Geometry: final body of the model. Coordinates: model frame, mm. Face numbers are marked on the shaded views. A direction names the side the tool comes from. Coordinates: 2 decimals unless noted, no trailing zeros. Write each loop counter-clockwise with the first axis right and the second up, starting at its lowest first coordinate (ties: lowest second). Pieces come first, ordered by that corner, then holes. Notation, with made-up numbers: (77, 56) - (87, 56) arc R9 cw to (87, 62) - close; hole circle Ø9 at (-27, 14.25). An arc over 180 degrees is marked (long way). Answer as a JSON object with one key per item and string values. Group by question number.
Item 1: Section D-D on y = -7.5. Return loops of the section in (x, z).
Item 2: Set-up query: the marked faces 1, 2 and 3. Return all of +Z, -Z, +X, -X, +Y, -Y with unobstructed straight access to the full face (end or side cutting, diameter ignored); none if empty.
Item 3: First-contact query: pin 1 Ø1 at (x, y) = (23.5, -0.5) entering from +Z; pin 2 Ø1 at (x, z) = (0, 5.5) entering from +Y; pin 3 Ø3.5 at (y, z) = (8.5, 3) entering from +X. Flat tips, straight axial feed; report the tip coordinate or a pass-through.
Item 4: Section A-A on y = 25.5. Return loops of the section in (x, z), and give its area (3 significant figures).
Item 5: Line query: line 1 along Z through (x, y) = (-2, -27); line 2 along Z through (x, y) = (6.5, 10.5); line 3 along X through (y, z) = (2.5, 8.5). Output: solid intervals per line, ascending. Write a range as from..to.
Item 6: Section B-B on z = 3.5. Return loops of the section in (x, y), and give its area (3 significant figures).
Item 7: Section C-C on x = -2.5. Return loops of the section in (y, z).
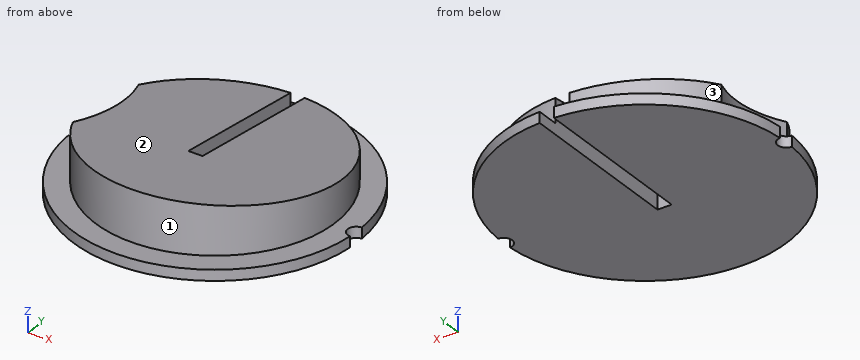
```python
from build123d import *

# Parameters (mm, degrees)
F1_DEPTH = 2.413
F3_DEPTH = 25.4
F5_DEPTH = 31.75
F7_DEPTH = 25.4


with BuildPart() as f1:
    # F0 (on Top) → F1 (new body)
    with BuildSketch(Plane.XY):
        with BuildLine():
            ThreePointArc((31.629235, -1.904139), (29.7815, 0), (31.629235, 1.904139))
            ThreePointArc((31.629235, 1.904139), (0, 31.6865), (-31.629235, 1.904139))
            ThreePointArc((-31.629235, 1.904139), (-29.7815, 0), (-31.629235, -1.904139))
            ThreePointArc((-31.629235, -1.904139), (0, -31.6865), (31.629235, -1.904139))
        make_face()
    extrude(amount=F1_DEPTH)

    # F2 (on face) → F3 (join)
    with BuildSketch(Plane.XY.offset(2.413)):
        with BuildLine():
            ThreePointArc((-24.485298, 10.571618), (-22.5425, 0), (-24.485298, -10.571618))
            ThreePointArc((-24.485298, -10.571618), (26.67, 0), (-24.485298, 10.571618))
        make_face()
    extrude(amount=F3_DEPTH)

    # F4 (on Right) → F5 (cut, symmetric)
    with BuildSketch(Plane.YZ):
        Polygon((-28.575, 36.80041), (-28.575, 13.97), (28.575, 7.62), (28.575, 36.80041), align=None)
    extrude(amount=F5_DEPTH, both=True, mode=Mode.SUBTRACT)

    # F6 (on face) → F7 (cut)
    with BuildSketch(Plane(origin=(0, 0, 0), x_dir=(1, 0, 0), z_dir=(0, 0, -1))):
        with BuildLine():
            Line((-1.5875, 6.2865), (-1.5875, -31.646708))
            ThreePointArc((-1.5875, -31.646708), (0, -31.6865), (1.5875, -31.646708))
            Line((1.5875, -31.646708), (1.5875, 6.2865))
            Line((1.5875, 6.2865), (-1.5875, 6.2865))
        make_face()
        with BuildLine():
            Line((-1.5875, -31.646708), (-1.5875, -44.5135))
            Line((-1.5875, -44.5135), (1.5875, -44.5135))
            Line((1.5875, -44.5135), (1.5875, -31.646708))
            ThreePointArc((1.5875, -31.646708), (0, -31.6865), (-1.5875, -31.646708))
        make_face()
    extrude(amount=-F7_DEPTH, mode=Mode.SUBTRACT)


solid = f1.part
```
Checks:
{
 "1": {"outline": "(-30.79, 0) - (30.79, 0) - (30.79, 2.41) - (25.59, 2.41) - (25.59, 11.63) - (-23.5, 11.63) - (-23.5, 2.41) - (-30.79, 2.41) - close"},
 "2": {"face 1": "+Z", "face 2": "+Z, +X, -X, +Y", "face 3": "+Z, -X, +Y"},
 "3": {"pin 1": "z = 10.91", "pin 2": "y = -6.29", "pin 3": "x = 30.94"},
 "4": {"outline": "(-18.81, 0) - (-1.59, 0) - (-1.59, 7.96) - (-7.81, 7.96) - (-7.81, 2.41) - (-18.81, 2.41) - close; (1.59, 0) - (18.81, 0) - (18.81, 2.41) - (7.81, 2.41) - (7.81, 7.96) - (1.59, 7.96) - close", "area": "152 mm^2"},
 "5": {"line 1": "0..2.41", "line 2": "0..9.63", "line 3": "-22.65..-1.59, 1.59..26.55"},
 "6": {"outline": "(-24.49, -10.57) arc R26.67 ccw (long way) to (1.59, 26.62) - (1.59, -6.29) - (-1.59, -6.29) - (-1.59, 26.62) arc R26.67 ccw to (-24.49, 10.57) arc R29.73 cw to start", "area": "2,070 mm^2"},
 "7": {"outline": "(-31.59, 0) - (31.59, 0) - (31.59, 2.41) - (26.55, 2.41) - (26.55, 7.84) - (-26.55, 13.75) - (-26.55, 2.41) - (-31.59, 2.41) - close"}
}
